Design review of the part built by this model. Coordinates are the model's own, in mm. A direction names the side the tool comes from. Round coordinates to 2 decimals unless told otherwise and drop trailing zeros. Loops run counter-clockwise (first coordinate to the right, second up) from the corner with the lowest first, then second, coordinate; pieces in that order, holes last. Notation, with made-up numbers: (-32.5, -20.75) - (-13.5, -20.75) arc R20 ccw to (-13.5, -2.75) - close; hole circle Ø9 at (20.25, 0.5). An arc over 180 degrees is marked (long way). Return JSON: item names as keys, results as strings. Group by question number.
(1) We need section C-C, the plane x = -87. Write out the cut boundary in (y, z), and give its area (3 significant figures).
(2) The part is to be moulded in two halves that separate along X. For faces 3 (the flat face through (-10.31, -27.605, 12.325)), 4 (the flat face through (-27.09, -19.56, 12.32)), 5 (the cylindrical face through (-106.543, 0.77, 12.325)), 6 (the flat face through (18.228, -14.086, 12.325)), say which applies: pulls with the +X half, pulls with the -X half, needs draft (parallel to the pull), parting line crosses it, or undercut.
(3) Wall thickness on L1, parallel to Y at x = -39.5, z = 2.75; L2, parallel to Y at x = -72, z = 14.75; L3, parallel to Y at x = 50, z = 1.75: over which ranges is each line inside the solid? List them lowest first. Write a range as [from, to].
(4) We need section B-B, the plane z = 7.25. Write out the cut boundary in (x, y).
(5) We need section D-D, the plane x = -42. Write out the cut boundary in (y, z).
(6) For faces 1 (the flat face through (-8.6, 27.4, 12.3)), 2 (the flat face through (-27.56, 19.615, 12.325)), list the 3-axis set-ups (+Z, -Z, +X, -X, +Y, -Y) from which the entire face can be reached by the end or side of a thin tool; tool diameter is ignored.
(7) Clearance check with flat-ended pins moving along their axes: pin 1 (6 mm diameter, centred on x = -60.5, z = 16, fed in from -Y); pin 2 (1.5 mm diameter, centred on x = -36, z = 9, fed in from -Y); pin 3 (6 mm diameter, centred on y = 21, z = 19.5, fed in from +X); pin 4 (18 mm diameter, centred on x = 52.67, y = 0, fed in from +Z). State where each tip first meets the part, or that it passes through.
(8) We need section A-A, the plane y = 0. Write out the cut boundary in (x, z).
from build123d import *

# Parameters (mm, degrees)
F0_R     = 25
F0_R_2   = 15
F1_DEPTH = 25


with BuildPart() as f1:
    # F0 (on Top) → F1 (new body)
    with BuildSketch(Plane.XY):
        with BuildLine():
            Line((52.66999, 20), (-71.551683, 35))
            ThreePointArc((-71.551683, 35), (-106.551683, 0), (-71.551683, -35))
            Line((-71.551683, -35), (52.66999, -20))
            ThreePointArc((52.66999, -20), (72.66999, 0), (52.66999, 20))
        make_face()
        with Locations((-71.551683, 0)):
            Circle(F0_R, mode=Mode.SUBTRACT)
        with BuildLine():
            ThreePointArc((-44.01352, -21.602074), (-36.551683, 0), (-44.01352, 21.602074))
            Line((-44.01352, 21.602074), (-10.639657, 17.572117))
            Line((-10.639657, 17.572117), (-10.639657, -17.572117))
            Line((-10.639657, -17.572117), (-44.01352, -21.602074))
        make_face(mode=Mode.SUBTRACT)
        with BuildLine():
            Line((-0.639657, 16.364599), (36.57403, 11.870976))
            ThreePointArc((36.57403, 11.870976), (32.66999, 0), (36.57403, -11.870976))
            Line((36.57403, -11.870976), (-0.639657, -16.364599))
            Line((-0.639657, -16.364599), (-0.639657, 16.364599))
        make_face(mode=Mode.SUBTRACT)
        with Locations((52.66999, 0)):
            Circle(F0_R_2, mode=Mode.SUBTRACT)
    extrude(amount=F1_DEPTH)


solid = f1.part
Solutions:
{
 "1": {"outline": "(-31.41, 0) - (-19.66, 0) - (-19.66, 25) - (-31.41, 25) - close; (19.66, 0) - (31.41, 0) - (31.41, 25) - (19.66, 25) - close", "area": "588 mm^2"},
 "2": {"face 3": "pulls with the +X half", "face 4": "undercut", "face 5": "pulls with the -X half", "face 6": "undercut"},
 "3": {"L1": "[-31.13, -21.06], [-14.06, 14.06], [21.06, 31.13]", "L2": "[-35, -25], [25, 35]", "L3": "[-20.32, -14.76], [14.76, 20.32]"},
 "4": {"outline": "(-71.55, -35) - (52.67, -20) arc R20 ccw to (52.67, 20) - (-71.55, 35) arc R35 ccw to start; hole circle Ø50 at (-71.55, 0); hole (-44.01, -21.6) - (-10.64, -17.57) - (-10.64, 17.57) - (-44.01, 21.6) arc R35 cw to start; hole (-0.64, -16.36) - (36.57, -11.87) arc R20 cw to (36.57, 11.87) - (-0.64, 16.36) - close; hole circle Ø30 at (52.67, 0)"},
 "5": {"outline": "(-31.43, 0) - (-21.36, 0) - (-21.36, 25) - (-31.43, 25) - close; (-18.75, 0) - (18.75, 0) - (18.75, 25) - (-18.75, 25) - close; (21.36, 0) - (31.43, 0) - (31.43, 25) - (21.36, 25) - close"},
 "6": {"face 1": "+Z, -Z, +X, +Y", "face 2": "+Z, -Z"},
 "7": {"pin 1": "y = -34.03", "pin 2": "y = -30.8", "pin 3": "x = 61.39", "pin 4": "through"},
 "8": {"outline": "(-106.55, 0) - (-96.55, 0) - (-96.55, 25) - (-106.55, 25) - close; (-46.55, 0) - (-36.55, 0) - (-36.55, 25) - (-46.55, 25) - close; (-10.64, 0) - (-0.64, 0) - (-0.64, 25) - (-10.64, 25) - close; (32.67, 0) - (37.67, 0) - (37.67, 25) - (32.67, 25) - close; (67.67, 0) - (72.67, 0) - (72.67, 25) - (67.67, 25) - close"}
}
